Geometry: final body of the model. Coordinates: model frame, mm. Face numbers are marked on the shaded views. Round coordinates to 2 decimals unless told otherwise and drop trailing zeros. Loops run counter-clockwise (first coordinate to the right, second up) from the corner with the lowest first, then second, coordinate; pieces in that order, holes last. Notation, with made-up numbers: (43, 8.25) - (47, 8.25) arc R11 ccw to (47, 22.25) - close; hole circle Ø7 at (-38.5, 65.5). An arc over 180 degrees is marked (long way). Write item = value, one per line. Start each with the question number.
Item 1: Draft query along Z for the marked faces 1, 2, 3 and 4. Return one class per face: pulls with the +Z half, pulls with the -Z half, needs draft (parallel to the pull), parting line crosses it, or undercut.
Item 2: Line query: line 1 (X direction, y = 3.25, z = -18); line 2 (X direction, y = 6.75, z = 0); line 3 (Z direction, x = -8, y = 4). Output: solid intervals per line, ascending. Write a range as from..to.
Item 3: Section B-B (x = 20). Return loops of the section in (y, z).
Item 4: Section D-D (y = 8). Count the separate pieces of the cut face and the enclosed holes in it, plus the area to 3 significant figures.
Item 5: Section A-A (z = -23). Return loops of the section in (x, y).
Item 6: Section C-C (z = 0). Return loops of the section in (x, y), plus the area to 3 significant figures.
from build123d import *

# Parameters (mm, degrees)
SKETCH_1_R          = 5.3
SKETCH_1_R_2        = 1.65
SKETCH_1_R_3        = 7.55
SKETCH_1_R_4        = 1.25
EXTRUDE_1_DEPTH     = 10
SKETCH_2_R          = 1.7
CUT_EXTRUDE_1_DEPTH = 10


with BuildPart() as part:
    # 草图1 → 凸台-拉伸1 (new body)
    with BuildSketch(Plane(origin=(0, 0, 0), x_dir=(1, 0, 0), z_dir=(0, 1, 0))):
        with BuildLine():
            Line((-35, 33), (35, 33))
            ThreePointArc((35, 33), (38.535533906, 31.535533906), (40, 28))
            Line((40, 28), (40, -15))
            ThreePointArc((40, -15), (38.535533906, -18.535533906), (35, -20))
            Line((35, -20), (-35, -20))
            ThreePointArc((-35, -20), (-38.535533906, -18.535533906), (-40, -15))
            Line((-40, -15), (-40, 28))
            ThreePointArc((-40, 28), (-38.535533906, 31.535533906), (-35, 33))
        make_face()
        Circle(SKETCH_1_R, mode=Mode.SUBTRACT)
        with Locations((0, 8)):
            Circle(SKETCH_1_R_2, mode=Mode.SUBTRACT)
        with Locations((8, 0)):
            Circle(SKETCH_1_R_2, mode=Mode.SUBTRACT)
        with Locations((0, -8)):
            Circle(SKETCH_1_R_2, mode=Mode.SUBTRACT)
        with Locations((-8, 0)):
            Circle(SKETCH_1_R_2, mode=Mode.SUBTRACT)
        with Locations((-25, 0)):
            Circle(SKETCH_1_R_3, mode=Mode.SUBTRACT)
        with Locations((-33.485281374, 8.485281374)):
            Circle(SKETCH_1_R_2, mode=Mode.SUBTRACT)
        with Locations((-16.514718626, 8.485281374)):
            Circle(SKETCH_1_R_2, mode=Mode.SUBTRACT)
        with Locations((-16.514718626, -8.485281374)):
            Circle(SKETCH_1_R_2, mode=Mode.SUBTRACT)
        with Locations((-33.485281374, -8.485281374)):
            Circle(SKETCH_1_R_2, mode=Mode.SUBTRACT)
        with Locations((25, 0)):
            Circle(SKETCH_1_R_3, mode=Mode.SUBTRACT)
        with Locations((16.514718626, 8.485281374)):
            Circle(SKETCH_1_R_2, mode=Mode.SUBTRACT)
        with Locations((16.514718626, -8.485281374)):
            Circle(SKETCH_1_R_2, mode=Mode.SUBTRACT)
        with Locations((33.485281374, -8.485281374)):
            Circle(SKETCH_1_R_2, mode=Mode.SUBTRACT)
        with Locations((33.485281374, 8.485281374)):
            Circle(SKETCH_1_R_2, mode=Mode.SUBTRACT)
        with Locations((-20, 23)):
            Circle(SKETCH_1_R_4, mode=Mode.SUBTRACT)
        with Locations((20, 23)):
            Circle(SKETCH_1_R_4, mode=Mode.SUBTRACT)
        with Locations((-29, 23)):
            Circle(SKETCH_1_R_4, mode=Mode.SUBTRACT)
        with Locations((29, 23)):
            Circle(SKETCH_1_R_4, mode=Mode.SUBTRACT)
    extrude(amount=EXTRUDE_1_DEPTH)

    # 草图2 → 切除-拉伸1 (cut)
    with BuildSketch(Plane(origin=(0, 10, 0), x_dir=(1, 0, 0), z_dir=(0, 1, 0))):
        with Locations((-9, 18)):
            Circle(SKETCH_2_R)
        with Locations((9, 18)):
            Circle(SKETCH_2_R)
    extrude(amount=-CUT_EXTRUDE_1_DEPTH, mode=Mode.SUBTRACT)


solid = part.part
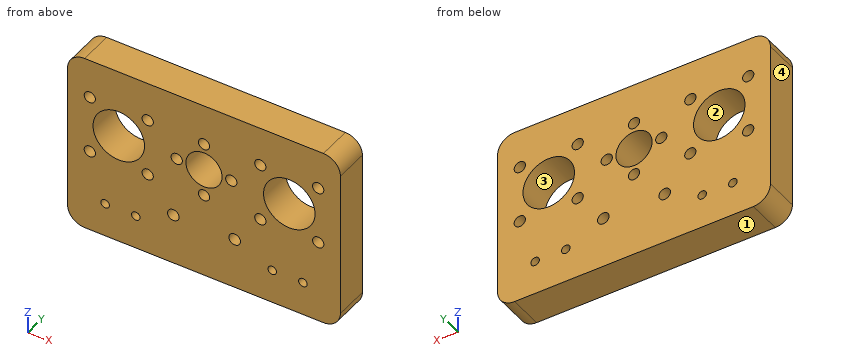
Taken from the geometry:
q1.face_1 = pulls with the -Z half
q1.face_2 = undercut
q1.face_3 = undercut
q1.face_4 = needs draft
q2.line_1 = -40..-10.7, -7.3..7.3, 10.7..40
q2.line_2 = -40..-32.55, -17.45..-9.65, -6.35..-5.3, 5.3..6.35, 9.65..17.45, 32.55..40
q2.line_3 = -33..-19.37, -16.63..-1.65, 1.65..20
q3.outline = (0, -33) - (10, -33) - (10, -24.25) - (0, -24.25) - close; (0, -21.75) - (10, -21.75) - (10, -5.66) - (0, -5.66) - close; (0, 5.66) - (10, 5.66) - (10, 20) - (0, 20) - close
q4.separate_pieces = 1
q4.enclosed_holes = 21
q4.area = 3,630 mm^2
q5.outline = (-40, 0) - (-30.25, 0) - (-30.25, 10) - (-40, 10) - close; (-27.75, 0) - (-21.25, 0) - (-21.25, 10) - (-27.75, 10) - close; (-18.75, 0) - (18.75, 0) - (18.75, 10) - (-18.75, 10) - close; (21.25, 0) - (27.75, 0) - (27.75, 10) - (21.25, 10) - close; (30.25, 0) - (40, 0) - (40, 10) - (30.25, 10) - close
q6.outline = (-40, 0) - (-32.55, 0) - (-32.55, 10) - (-40, 10) - close; (-17.45, 0) - (-9.65, 0) - (-9.65, 10) - (-17.45, 10) - close; (-6.35, 0) - (-5.3, 0) - (-5.3, 10) - (-6.35, 10) - close; (5.3, 0) - (6.35, 0) - (6.35, 10) - (5.3, 10) - close; (9.65, 0) - (17.45, 0) - (17.45, 10) - (9.65, 10) - close; (32.55, 0) - (40, 0) - (40, 10) - (32.55, 10) - close
q6.area = 326 mm^2
